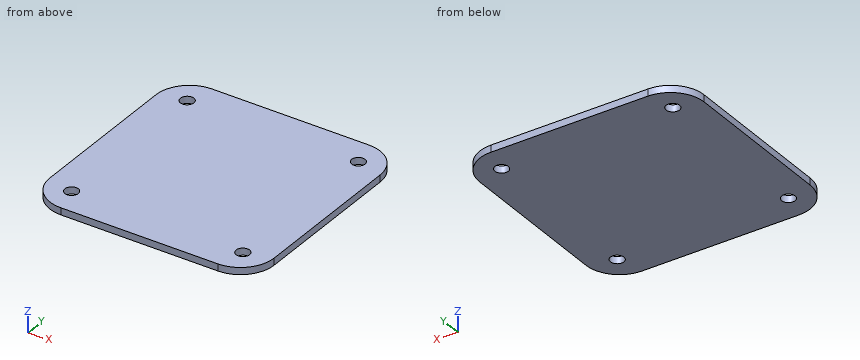
```python
from build123d import *

# Parameters (mm, degrees)
SKETCH1_W           = 100
SKETCH1_H           = 100
SKETCH1_R           = 3
BOSS_EXTRUDE2_DEPTH = 3.1
FILLET1_R           = 15


with BuildPart() as part:
    # Sketch1 → Boss-Extrude2 (new body)
    with BuildSketch(Plane.XY):
        Rectangle(SKETCH1_W, SKETCH1_H)
        with Locations((-38.166088515, 38.166088515)):
            Circle(SKETCH1_R, mode=Mode.SUBTRACT)
        with Locations((38.166088515, 38.166088515)):
            Circle(SKETCH1_R, mode=Mode.SUBTRACT)
        with Locations((38.166088515, -38.166088515)):
            Circle(SKETCH1_R, mode=Mode.SUBTRACT)
        with Locations((-38.166088515, -38.166088515)):
            Circle(SKETCH1_R, mode=Mode.SUBTRACT)
    extrude(amount=BOSS_EXTRUDE2_DEPTH)

    # Fillet1
    fillet1_edges = [part.edges().sort_by_distance(p)[0] for p in [
        (50, -50, 1.55),
        (-50, -50, 1.55),
        (-50, 50, 1.55),
        (50, 50, 1.55),
    ]]
    fillet(fillet1_edges, radius=FILLET1_R)


solid = part.part
```
The model under review builds one solid part; all positions refer to its coordinate system, in mm. Round coordinates to 2 decimals unless told otherwise and drop trailing zeros. Loops run counter-clockwise (first coordinate to the right, second up) from the corner with the lowest first, then second, coordinate; pieces in that order, holes last. Notation, with made-up numbers: (86.25, -35) -> (116.25, -35) arc R22 ccw to (116.25, -18) -> close; hole circle Ø10 at (0, 30). An arc over 180 degrees is marked (long way). Answer in a Markdown table with one row per item.
1) Consider section A-A, the plane z = 1.3. Write out the cut boundary in (x, y), plus the area to 3 significant figures.
Taken from the geometry:
| item | result |
|---|---|
| outline | (-50, -35) arc R15 ccw to (-35, -50) -> (35, -50) arc R15 ccw to (50, -35) -> (50, 35) arc R15 ccw to (35, 50) -> (-35, 50) arc R15 ccw to (-50, 35) -> close; hole circle Ø6 at (-38.17, -38.17); hole circle Ø6 at (-38.17, 38.17); hole circle Ø6 at (38.17, -38.17); hole circle Ø6 at (38.17, 38.17) |
| area | 9,690 mm² |
2) Wall thickness on line 1 along X through (y, z) = (-37.5, 2.3); line 2 along Y through (x, z) = (39, 1.25): over which ranges is each line inside the solid? List them lowest first.
Taken from the geometry:
| item | result |
|---|---|
| line 1 | x = -49.79 to -41.09, -35.24 to 35.24, 41.09 to 49.79 |
| line 2 | y = -49.46 to -41.05, -35.28 to 35.28, 41.05 to 49.46 |
3) Consider section B-B, the plane y = -43. Write out the cut boundary in (x, z), plus the area to 3 significant figures.
Taken from the geometry:
| item | result |
|---|---|
| outline | (-47.69, 0) -> (47.69, 0) -> (47.69, 3.1) -> (-47.69, 3.1) -> close |
| area | 296 mm² |
